Read the model definition and answer for the solid it produces. Units are mm, in the model's axes. Coordinates: 2 decimals unless noted, no trailing zeros. Write each loop counter-clockwise with the first axis right and the second up, starting at its lowest first coordinate (ties: lowest second). Pieces come first, ordered by that corner, then holes. Notation, with made-up numbers: (-19, 1) -> (4, 1) arc R37 cw to (4, 38) -> close; hole circle Ø9 at (42.25, -30.5). An arc over 180 degrees is marked (long way). Answer in a Markdown table with one row per item. Add a question column.
Item 1: Section B-B on z = 308.5 is taken. Write down the section's boundary in (x, y) (3 decimals).
Item 2: Section A-A on y = -359.5 is taken. Write down the section's boundary in (x, z) (3 decimals).
Item 3: Straight lines are drawn through the part: line 1 (Z direction, x = 308, y = -448.5) (3 decimals); line 2 (X direction, y = -155.5, z = 238) (3 decimals); line 3 (X direction, y = -219, z = 313) (3 decimals). For each, find the intervals that lie inside material, in ascending order. Write a range as from..to.
```python
from build123d import *

# Parameters (mm, degrees)
F0_W     = 361.95
F0_H     = 692.15
F1_DEPTH = 581.025
F2_W     = 330.2
F2_H     = 660.4
F3_DEPTH = 565.15
F4_W     = 325.12
F4_H     = 655.32
F5_DEPTH = 565.15
F7_DEPTH = 565.15


with BuildPart() as f1:
    # F0 (on Front) → F1 (new body)
    with BuildSketch(Plane.XZ):
        with Locations((180.975, 346.075)):
            Rectangle(F0_W, F0_H)
    extrude(amount=F1_DEPTH)

    # F2 (on face) → F3 (cut)
    with BuildSketch(Plane.XZ.offset(581.025)):
        with Locations((180.975, 346.075)):
            Rectangle(F2_W, F2_H)
    extrude(amount=-F3_DEPTH, mode=Mode.SUBTRACT)

    # F4 (on face) → F5 (join)
    with BuildSketch(Plane.XZ.offset(581.025)):
        with Locations((180.975, 346.075)):
            Rectangle(F4_W, F4_H)
    extrude(amount=-F5_DEPTH)

    # F6 (on face) → F7 (cut)
    with BuildSketch(Plane.XZ.offset(581.025)):
        Polygon((37.465, 400.05), (18.415, 431.8), (18.415, 266.7), (37.465, 298.45), align=None)
    extrude(amount=-F7_DEPTH, mode=Mode.SUBTRACT)


solid = f1.part
```
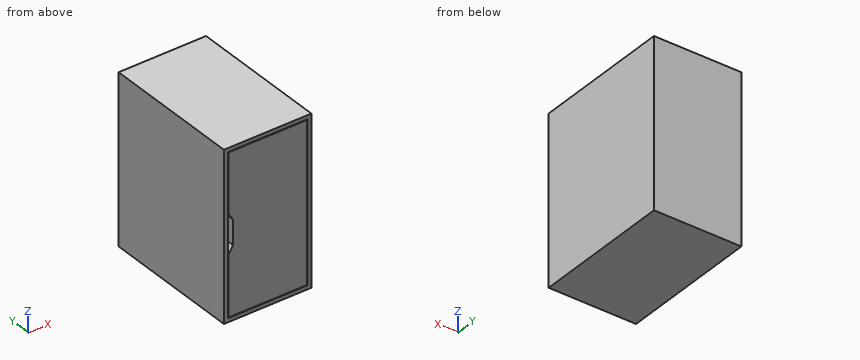
Results below:
| question | item | result |
|---|---|---|
| 1 | outline | (0, -581.025) -> (15.875, -581.025) -> (15.875, -15.875) -> (37.465, -15.875) -> (37.465, -581.025) -> (343.535, -581.025) -> (343.535, -15.875) -> (346.075, -15.875) -> (346.075, -581.025) -> (361.95, -581.025) -> (361.95, 0) -> (0, 0) -> close |
| 2 | outline | (0, 0) -> (361.95, 0) -> (361.95, 692.15) -> (0, 692.15) -> close; (18.415, 18.415) -> (343.535, 18.415) -> (343.535, 673.735) -> (18.415, 673.735) -> (18.415, 431.8) -> (37.465, 400.05) -> (37.465, 298.45) -> (18.415, 266.7) -> close; hole (15.875, 15.875) -> (346.075, 15.875) -> (346.075, 676.275) -> (15.875, 676.275) -> close |
| 3 | line 1 | z = 0..15.875, 18.415..673.735, 676.275..692.15 |
| 3 | line 2 | x = 0..15.875, 18.415..343.535, 346.075..361.95 |
| 3 | line 3 | x = 0..15.875, 37.465..343.535, 346.075..361.95 |
